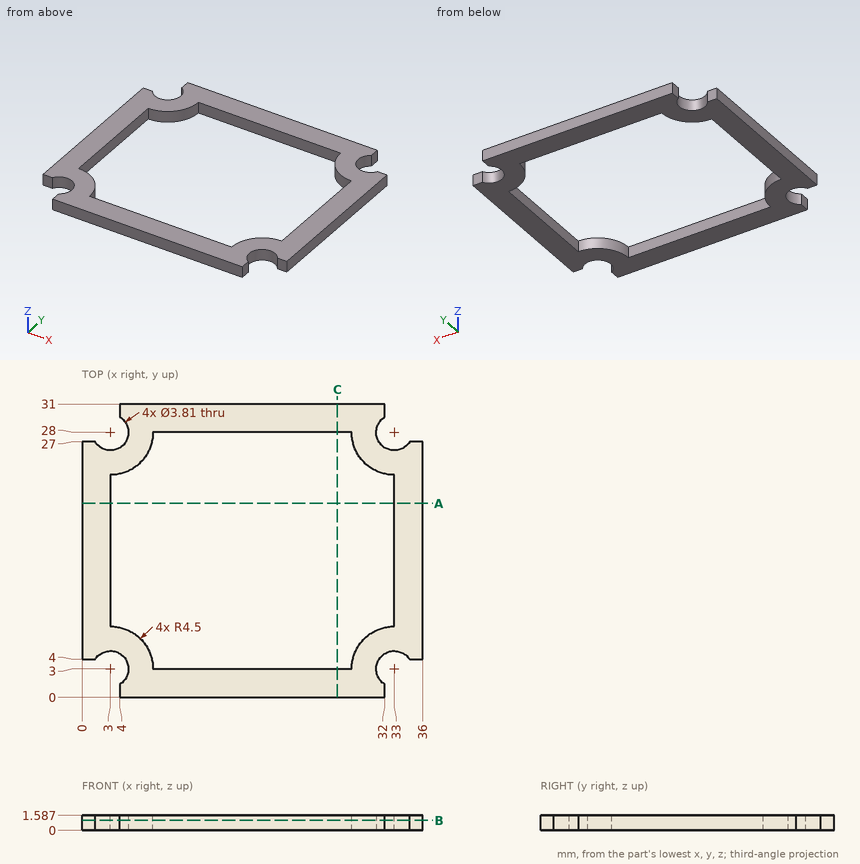
For this review, use the dimensioned drawing (mm, ordinates from the lowest corner) and the shaded views. Coordinates: 2 decimals unless noted, no trailing zeros. Write each loop counter-clockwise with the first axis right and the second up, starting at its lowest first coordinate (ties: lowest second). Pieces come first, ordered by that corner, then holes. Notation, with made-up numbers: (3.5, 2) - (41.5, 2) arc R21 cw to (41.5, 41) - close; hole circle Ø1 at (44.25, -5). An arc over 180 degrees is marked (long way). Answer in a Markdown table with one row per item. Add a question column.
Q1. Consider section A-A on y = 20.5. Give the boundary of the cut face in (x, z).
Q2. Consider section B-B on z = 1.05. Give the boundary of the cut face in (x, y) (1 decimal), then the cut area to 3 significant figures.
Q3. To check wall thickness, follow line 1 along X through (y, z) = (13.5, 0.4); line 2 along Y through (x, z) = (20, 0.8); line 3 along X through (y, z) = (25.5, 1.4). State the ranges of each line that lie inside material, in increasing order. Write a range as from..to.
Q4. Consider section C-C on x = 27. Give the boundary of the cut face in (y, z).
Q5. Clearance check with flat-ended pins moving along their axes: pin 1 (0.7 mm diameter, centred on x = 1, z = 1, fed in from -Y); pin 2 (0.7 mm diameter, centred on y = 0.5, z = 0.5, fed in from +X). State where each tip first meets the part, or that it passes through.
Answers below:
| question | item | result |
|---|---|---|
| 1 | outline | (0, 0) - (3, 0) - (3, 1.59) - (0, 1.59) - close; (33, 0) - (36, 0) - (36, 1.59) - (33, 1.59) - close |
| 2 | outline | (0, 4) - (1.4, 4) arc R1.9 cw (long way) to (4, 1.4) - (4, 0) - (32, 0) - (32, 1.4) arc R1.9 cw (long way) to (34.6, 4) - (36, 4) - (36, 27) - (34.6, 27) arc R1.9 cw (long way) to (32, 29.6) - (32, 31) - (4, 31) - (4, 29.6) arc R1.9 cw (long way) to (1.4, 27) - (0, 27) - close; hole (3, 7.5) arc R4.5 cw to (7.5, 3) - (28.5, 3) arc R4.5 cw to (33, 7.5) - (33, 23.5) arc R4.5 cw to (28.5, 28) - (7.5, 28) arc R4.5 cw to (3, 23.5) - close |
| 2 | area | 350 mm² |
| 3 | line 1 | 0..3, 33..36 |
| 3 | line 2 | 0..3, 28..31 |
| 3 | line 3 | 0..6.74, 29.26..36 |
| 4 | outline | (0, 0) - (3, 0) - (3, 1.59) - (0, 1.59) - close; (28, 0) - (31, 0) - (31, 1.59) - (28, 1.59) - close |
| 5 | pin 1 | y = 4 |
| 5 | pin 2 | x = 32 |
